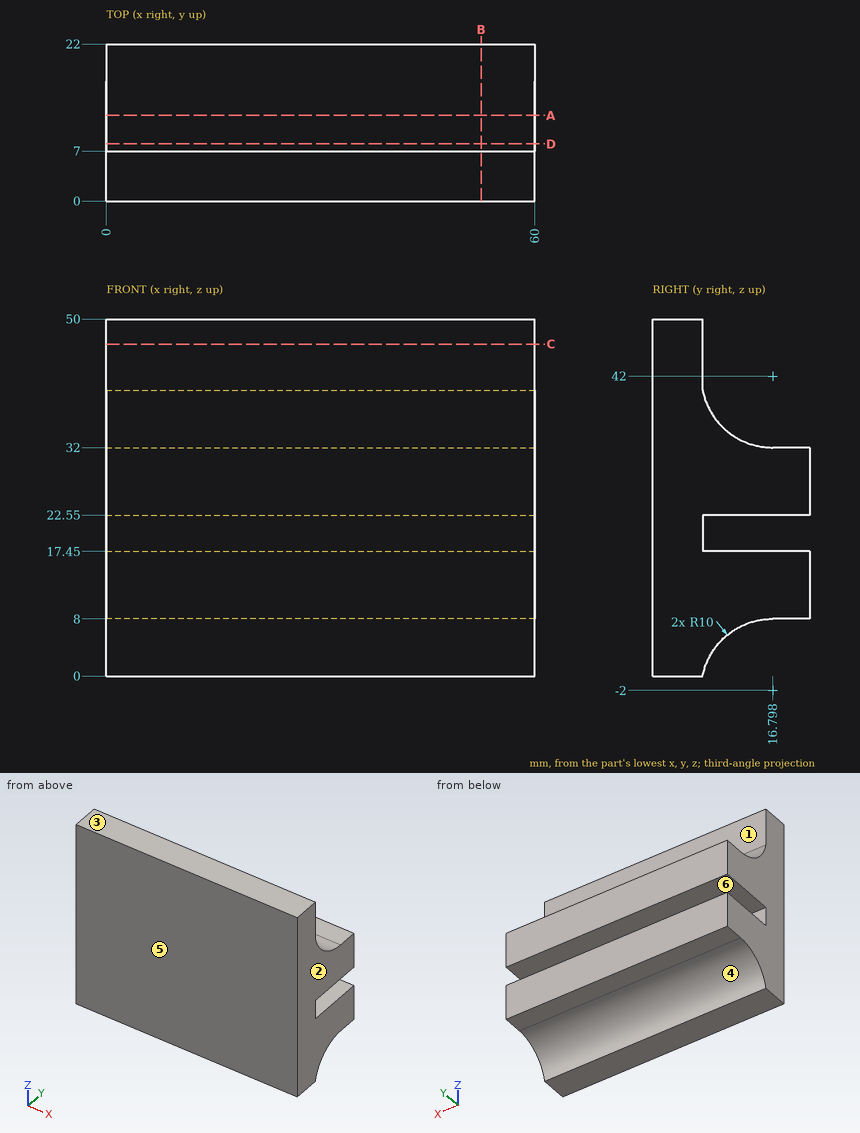
Print and shaded views of the part. All mm, measured from the part's lowest x, y and z. A direction names the side the tool comes from. Coordinates: 2 decimals unless noted, no trailing zeros. Write each loop counter-clockwise with the first axis right and the second up, starting at its lowest first coordinate (ties: lowest second). Pieces come first, ordered by that corner, then holes. Notation, with made-up numbers: (-32.75, 82.5) -> (-23.75, 82.5) arc R4 cw to (-23.75, 88.5) -> close; hole circle Ø9 at (26.25, 60.5). An arc over 180 degrees is marked (long way). Use CSV: the item, a comma, the result in double quotes. Start each with the question number.
Q1. Cut at D-D, the plane y = 8. List the corners of the cut face in (x, z), then the cut area to 3 significant figures.
Q2. Cut at C-C, the plane z = 46.5. List the corners of the cut face in (x, y).
Q3. Cut at A-A, the plane y = 12. List the corners of the cut face in (x, z).
Q4. Cut at B-B, the plane x = 52.5. List the corners of the cut face in (y, z), then the cut area to 3 significant figures.
Q5. Pull direction Z, two halves, no side cores. Call the marked faces 3, 4, 5 and 6: released by +Z, released by -Z, zero draft, split by the parting line, or undercut.
Q6. 3-axis set-ups, long thin cutter, end or side, ignore diameter. For the marked faces 1 and 2: which of +Z, -Z, +X, -X, +Y, -Y reach the whole face in a straight line?
Q7. Drill centre lines: probe 1 along Z at (x, y) = (37, 20); probe 2 along Y at (x, z) = (33.5, 18); probe 3 along Z at (x, y) = (15.5, 14). Where is each one in solid material? Low to high.
Q8. Flat gauge pins, fed straight in: pin 1 Ø1.6 at (x, y) = (36.5, 20) entering from -Z; pin 2 Ø10 at (y, z) = (14.5, 35.5) entering from -X; pin 3 Ø5 at (x, y) = (9, 10.5) entering from -Z; pin 4 Ø7.5 at (x, y) = (19, 18) entering from -Z. Where does each tip first touch, or does it go through?
Checked values:
1,outline,"(0, 2.75) -> (60, 2.75) -> (60, 17.45) -> (0, 17.45) -> close; (0, 22.55) -> (60, 22.55) -> (60, 37.25) -> (0, 37.25) -> close"
1,area,"1,760 mm²"
2,outline,"(0, 0) -> (60, 0) -> (60, 7) -> (0, 7) -> close"
3,outline,"(0, 6.77) -> (60, 6.77) -> (60, 17.45) -> (0, 17.45) -> close; (0, 22.55) -> (60, 22.55) -> (60, 33.23) -> (0, 33.23) -> close"
4,outline,"(0, 0) -> (7, 0) arc R10 cw to (16.8, 8) -> (22, 8) -> (22, 17.45) -> (7, 17.45) -> (7, 22.55) -> (22, 22.55) -> (22, 32) -> (16.8, 32) arc R10 cw to (7, 40) -> (7, 50) -> (0, 50) -> close"
4,area,"673 mm²"
5,face 3,"released by +Z"
5,face 4,"released by -Z"
5,face 5,"zero draft"
5,face 6,"undercut"
6,face 1,"+Z, +X, -X, +Y"
6,face 2,"+Z, -Z, +X, +Y, -Y"
7,probe 1,"z = 8 to 17.45, 22.55 to 32"
7,probe 2,"y = 0 to 7"
7,probe 3,"z = 7.6 to 17.45, 22.55 to 32.4"
8,pin 1,"stops at z = 8"
8,pin 2,"stops at x = 0"
8,pin 3,"stops at z = 2.75"
8,pin 4,"stops at z = 7.67"
